Verification items for the finished model (mm, model axes). Face numbers are marked on the shaded views. A direction names the side the tool comes from. Coordinates: 2 decimals unless noted, no trailing zeros. Order: outer loops, then holes, each group sorted by start corner. A loop starts at its lowest first (then second) coordinate and runs counter-clockwise, first axis right, second up. Notation, with made-up numbers: M -35.5,38 L -29.5,38 A28 ccw -29.5,76 Z; hole C 59,86.5 d7. An arc over 180 degrees is marked long. Return JSON: item names as keys, results as strings. Group by question number.
1. Section check D-D, the plane z = -10. Record the cut outline in (x, y).
2. Gauge pin test, flat ends, axial feed: pin 1 (4 mm diameter, centred on y = 23.5, z = 6, fed in from -X); pin 2 (1 mm diameter, centred on x = -5, y = 34, fed in from -Z); pin 3 (6 mm diameter, centred on x = -1, y = 46.5, fed in from -Z). Record the tip position at first contact, or that the pin passes through.
3. Section check C-C, the plane x = 9.75. Record the cut outline in (y, z).
4. Set-up check for the marked faces 5 and 6: record each of +Z, -Z, +X, -X, +Y, -Y from which the full face is reachable in a straight line by a thin tool's end or side.
5. Mould release check, pull along Y, two halves, no side actions. Record for the marked faces 1, 2, 3 and 4: +Y half, -Y half, draft (parallel to the pull), parting line (faces both ways), or undercut.
6. Section check B-B, the plane y = 60. Record the cut outline in (x, z), plus the area to 3 significant figures.
7. Section check A-A, the plane z = 7. Record the cut outline in (x, y).
8. Material ranges on line 1 along Z through (x, y) = (0, 3); line 2 along X through (y, z) = (6.75, 0), recorded low to high.
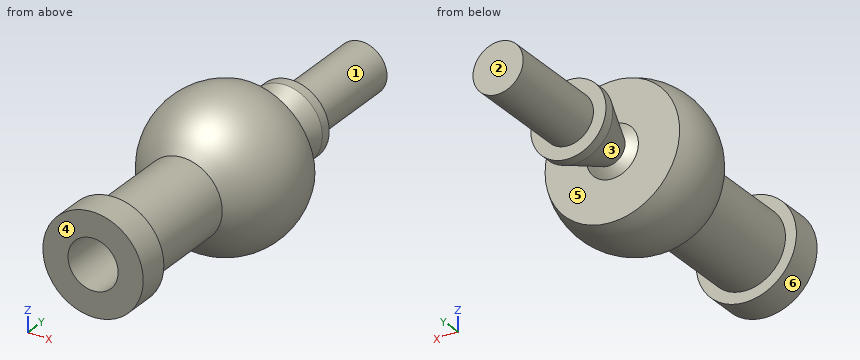
```python
from build123d import *


with BuildPart() as part:
    # 草图1 → 旋转1 (revolve)
    with BuildSketch(Plane.XY):
        with BuildLine():
            Line((0, 12.038127602), (4, 9.728726525))
            Line((4, 9.728726525), (4, 0))
            Line((4, 0), (8, 0))
            Line((8, 0), (8, 5))
            Line((8, 5), (6.25, 5))
            Line((6.25, 5), (6.25, 21.756099376))
            ThreePointArc((6.25, 21.756099376), (11.534904039, 28.691527723), (10.729508749, 37.373792144))
            Line((10.729508749, 37.373792144), (4.14914812, 37.373792144))
            ThreePointArc((4.14914812, 37.373792144), (3.412230956, 37.869391112), (2.616929575, 38.264563171))
            Line((2.616929575, 38.264563171), (6, 46.363160318))
            Line((6, 46.363160318), (6, 48))
            Line((6, 48), (4, 48))
            Line((4, 48), (4, 65))
            Line((4, 65), (0, 65))
            Line((0, 65), (0, 12.038127602))
        make_face()
    revolve(axis=Axis((0, 0.112242194, 0), (0, 1, 0)))


solid = part.part
```
Answers follow:
{
 "1": {"outline": "M -3.89,37.37 A6.63 ccw long 3.89,37.37 Z"},
 "2": {"pin 1": "x = -8.57", "pin 2": "z = -10.96", "pin 3": "z = -6"},
 "3": {"outline": "M 37.37,-4.48 L 37.37,4.48 A7 ccw long Z"},
 "4": {"face 5": "none", "face 6": "-Y"},
 "5": {"face 1": "draft", "face 2": "+Y half", "face 3": "undercut", "face 4": "-Y half"},
 "6": {"outline": "C 0,0 d8", "area": "50.3 mm^2"},
 "7": {"outline": "M -8.13,37.37 A9.75 ccw long 8.13,37.37 Z; M -3.87,0 L 3.87,0 L 3.87,5 L -3.87,5 Z"},
 "8": {"line 1": "-8 to -4, 4 to 8", "line 2": "-6.25 to -4, 4 to 6.25"}
}
